from build123d import *

# Parameters (mm, degrees)
SKETCH1_W           = 82.55
SKETCH1_H           = 69.85
BOSS_EXTRUDE1_DEPTH = 38.1
SKETCH2_R           = 5.159375
CUT_EXTRUDE2_DEPTH  = 115.652235041
SKETCH3_R           = 7.3421875
CUT_EXTRUDE3_DEPTH  = 28.448
SKETCH4_R           = 12.7254
CUT_EXTRUDE4_DEPTH  = 2.8194
SKETCH6_R           = 12.7254
CUT_EXTRUDE7_DEPTH  = 2.8194


with BuildPart() as part:
    # Sketch1 → Boss-Extrude1 (new body)
    with BuildSketch(Plane.YZ):
        with Locations((41.275, 34.925)):
            Rectangle(SKETCH1_W, SKETCH1_H)
    extrude(amount=BOSS_EXTRUDE1_DEPTH)

    # Sketch2 → Cut-Extrude2 (cut, through all)
    with BuildSketch(Plane.YZ):
        with Locations(Location((11.049, 11.049, 0), (0, 0, 270))):
            Circle(SKETCH2_R)
        with Locations(Location((71.374, 11.049, 0), (0, 0, 270))):
            Circle(SKETCH2_R)
        with Locations(Location((11.049, 58.674, 0), (0, 0, 270))):
            Circle(SKETCH2_R)
        with Locations(Location((71.374, 58.674, 0), (0, 0, 270))):
            Circle(SKETCH2_R)
    extrude(amount=CUT_EXTRUDE2_DEPTH, mode=Mode.SUBTRACT)

    # Sketch3 → Cut-Extrude3 (cut)
    with BuildSketch(Plane.YZ):
        with Locations(Location((23.622, 34.798, 0), (0, 0, 270))):
            Circle(SKETCH3_R)
        with Locations(Location((58.674, 34.798, 0), (0, 0, 270))):
            Circle(SKETCH3_R)
    extrude(amount=CUT_EXTRUDE3_DEPTH, mode=Mode.SUBTRACT)

    # Sketch4 → Cut-Extrude4 (cut)
    with BuildSketch(Plane.YZ):
        with Locations(Location((23.622, 34.798, 0), (0, 0, 270))):
            Circle(SKETCH4_R)
        with Locations(Location((58.674, 34.798, 0), (0, 0, 270))):
            Circle(SKETCH4_R)
    extrude(amount=CUT_EXTRUDE4_DEPTH, mode=Mode.SUBTRACT)

    # Sketch6 → Cut-Extrude7 (cut)
    with BuildSketch(Plane.YZ):
        with Locations((0, 41.275)):
            Circle(SKETCH6_R)
    extrude(amount=CUT_EXTRUDE7_DEPTH, mode=Mode.SUBTRACT)


solid = part.part
Verification items for the finished model (mm, model axes). A direction names the side the tool comes from. Give positions to 0.01 mm unless a question says otherwise; leave off trailing zeros. Loops run counter-clockwise (first coordinate to the right, second up) from the corner with the lowest first, then second, coordinate; pieces in that order, holes last.
1) Draft check along Y on faces 1 (the flat face through (19, 0, 34)), 2 (the flat face through (38.1, 41, 35)), 3 (the cylindrical face through (18.78, 6.01, 59.79)). Enter one of: pulls with the +Y half, pulls with the -Y half, needs draft (parallel to the pull), parting line crosses it, or undercut.
2) Thickness scan on line 1 along Y through (x, z) = (27, 15.5); line 2 along Y through (x, z) = (18, 9); line 3 along Z through (x, y) = (21.5, 74). Record the ranges inside material, lowest first.
3) Set-up check for faces 4 (the flat face through (19, 82.55, 34)), 5 (the cylindrical face through (15.454, 25.827, 27.795)), 6 (the cylindrical face through (1.39, 9.06, 50.21)): record each of +Z, -Z, +X, -X, +Y, -Y from which the full face is reachable in a straight line by a thin tool's end or side.
4) Sectioned sample at B-B, the plane x = 5.5. Enter the section's corners in (y, z), then the cut area to 3 significant figures.
5) Sectioned sample at D-D, the plane y = 32.5. Enter the section's corners in (x, z), then the cut area to 3 significant figures.
6) Depth check by flat-ended pin: pin 1 Ø13.5 at (y, z) = (11.049, 58.674) entering from -X; pin 2 Ø7.5 at (y, z) = (23, 38) entering from -X; pin 3 Ø9.5 at (y, z) = (71.374, 11.049) entering from +X; pin 4 Ø19 at (y, z) = (23.622, 34.798) entering from -X. Enter the tip coordinate at first touch or a pass-through.
7) Sectioned sample at A-A, the plane y = 73.5. Enter the section's corners in (x, z), then the cut area to 3 significant figures.
8) Sectioned sample at C-C, the plane z = 45. Enter the section's corners in (x, y), then the cut area to 3 significant figures.
Answers:
1. face 1: pulls with the -Y half
1. face 2: needs draft
1. face 3: undercut
2. line 1: y = 0 to 8.44, 13.66 to 68.76, 73.98 to 82.55
2. line 2: y = 0 to 6.31, 15.78 to 66.64, 76.11 to 82.55
2. line 3: z = 0 to 6.61, 15.49 to 54.23, 63.12 to 69.85
3. face 4: +Z, -Z, +X, -X, +Y
3. face 5: -X
3. face 6: -X, -Y
4. outline: (0, 0) - (82.55, 0) - (82.55, 69.85) - (0, 69.85) - close; hole circle Ø10.32 at (11.05, 11.05); hole circle Ø10.32 at (11.05, 58.67); hole circle Ø14.68 at (23.62, 34.8); hole circle Ø14.68 at (58.67, 34.8); hole circle Ø10.32 at (71.37, 11.05); hole circle Ø10.32 at (71.37, 58.67)
4. area: 5,090 mm2
5. outline: (0, 0) - (38.1, 0) - (38.1, 69.85) - (0, 69.85) - (0, 43.91) - (2.82, 43.91) - (2.82, 25.68) - (0, 25.68) - close
5. area: 2,610 mm2
6. pin 1: stops at x = 0
6. pin 2: stops at x = 28.45
6. pin 3: passes through
6. pin 4: stops at x = 2.82
7. outline: (0, 0) - (38.1, 0) - (38.1, 6.35) - (0, 6.35) - close; (0, 15.75) - (38.1, 15.75) - (38.1, 53.97) - (0, 53.97) - close; (0, 63.37) - (38.1, 63.37) - (38.1, 69.85) - (0, 69.85) - close
7. area: 1,940 mm2
8. outline: (0, 12.17) - (2.82, 12.17) - (2.82, 0) - (38.1, 0) - (38.1, 82.55) - (0, 82.55) - (0, 66.28) - (2.82, 66.28) - (2.82, 51.07) - (0, 51.07) - (0, 31.23) - (2.82, 31.23) - (2.82, 16.02) - (0, 16.02) - close
8. area: 3,030 mm2
